```python
from build123d import *

# Parameters (mm, degrees)
SKETCH1_W            = 107
SKETCH1_H            = 36.5
BATTERY_DEPTH        = 30
CABLES_DEPTH         = 10
CABLES_DEPTH_BACK    = 5
F_1MM_EDGE_FILLETS_R = 1


with BuildPart() as part:
    # Sketch1 → Battery (new body)
    with BuildSketch(Plane(origin=(0, 0, 0), x_dir=(1, 0, 0), z_dir=(0, 1, 0))):
        Rectangle(SKETCH1_W, SKETCH1_H)
    extrude(amount=BATTERY_DEPTH)

    # Sketch2 → Cables (add, two sides: drawn at the far end of the back side and taken through both)
    with BuildSketch(Plane.ZY.offset(53.5).offset(-CABLES_DEPTH_BACK)):
        with BuildLine():
            Line((-21.25, 9.5), (-21.25, 13.5))
            ThreePointArc((-21.25, 13.5), (-19.75, 15), (-18.25, 13.5))
            Line((-18.25, 13.5), (-18.25, 9.5))
            ThreePointArc((-18.25, 9.5), (-19.75, 8), (-21.25, 9.5))
        make_face()
        with BuildLine():
            Line((17.25, 8.5), (17.25, 14.5))
            ThreePointArc((17.25, 14.5), (18.25, 15.5), (19.25, 14.5))
            Line((19.25, 14.5), (19.25, 8.5))
            ThreePointArc((19.25, 8.5), (18.25, 7.5), (17.25, 8.5))
        make_face()
    extrude(amount=CABLES_DEPTH + CABLES_DEPTH_BACK)

    # 1mm Edge Fillets
    f_1mm_edge_fillets_edges = [part.edges().sort_by_distance(p)[0] for p in [
        (0, 0, 18.25),
        (0, 0, -18.25),
        (-53.5, 0, 0),
        (0, 30, -18.25),
        (0, 30, 18.25),
        (-53.5, 30, 0),
        (53.5, 15, 18.25),
        (53.5, 30, 0),
        (53.5, 15, -18.25),
        (53.5, 0, 0),
        (-53.5, 3.75, 18.25),
        (-53.5, 22.75, 18.25),
    ]]
    fillet(f_1mm_edge_fillets_edges, radius=F_1MM_EDGE_FILLETS_R - 0.0001)  # a hair under: the kernel refuses the full size


solid = part.part
```
Geometry check sheet. Reference: the model listing, model coordinates, mm. A direction names the side the tool comes from. Coordinates: 2 decimals unless noted, no trailing zeros. Loops run counter-clockwise (first coordinate to the right, second up) from the corner with the lowest first, then second, coordinate; pieces in that order, holes last. Notation, with made-up numbers: (-28, -15.5) - (-10, -15.5) arc R24 ccw to (-10, 23.5) - close; hole circle Ø2 at (50, 70). An arc over 180 degrees is marked (long way). One line per item, written item: value. Start each with the question number.
(1) Cross-section at D-D on z = -19.75. Enter the section's corners in (x, y), plus the area to 3 significant figures.
(2) Cross-section at C-C on z = 9. Enter the section's corners in (x, y).
(3) Cross-section at B-B on y = 26.5. Enter the section's corners in (x, z).
(4) Mould release check, pull along Z, two halves, no side actions. Record for faces 5 (the flat face through (-1, 15, 18.25)), 6 (the flat face through (-58, 11, 17.25)), 7 (the flat face through (-48.5, 12, -20)): released by +Z, released by -Z, zero draft, split by the parting line, or undercut.
(5) Cross-section at A-A on x = -29.5. Enter the section's corners in (y, z).
(6) Tool access check on faces 1 (the cylindrical face through (-57.562, 7.568, 18.613)), 2 (the flat face through (-1, 30, 0)), 3 (the flat face through (-58, 12, -18.25)), 4 (the cylindrical face through (-57.562, 15.447, 18.571)). Record the directions out of +Z, -Z, +X, -X, +Y, -Y that give a thin tool (end or side, any length) a straight path to the whole face; none if there is none.
(7) Material ranges on line 1 (X direction, y = 12.5, z = 13); line 2 (Z direction, x = 20.5, y = 8), recorded low to high. Write a range as [from, to].
(8) Depth check by flat-ended pin: P1, Ø6, axis at x = -24, y = 17.5, coming from the +Z side; P2, Ø14, axis at y = 21, z = -6, coming from the -X side; P3, Ø5, axis at x = -13.5, y = 17.5, coming from the -Z side. Enter the tip coordinate at first touch or a pass-through.
Results below:
1. outline: (-63.5, 8) - (-48.5, 8) - (-48.5, 15) - (-63.5, 15) - close
1. area: 105 mm2
2. outline: (-53.5, 1) arc R1 ccw to (-52.5, 0) - (52.5, 0) arc R1 ccw to (53.5, 1) - (53.5, 29) arc R1 ccw to (52.5, 30) - (-52.5, 30) arc R1 ccw to (-53.5, 29) - close
3. outline: (-53.5, -18.25) - (52.5, -18.25) arc R1 ccw to (53.5, -17.25) - (53.5, 17.25) arc R1 ccw to (52.5, 18.25) - (-52.5, 18.25) arc R1 ccw to (-53.5, 17.25) - close
4. face 5: released by +Z
4. face 6: undercut
4. face 7: zero draft
5. outline: (0, -17.25) arc R1 ccw to (1, -18.25) - (29, -18.25) arc R1 ccw to (30, -17.25) - (30, 17.25) arc R1 ccw to (29, 18.25) - (1, 18.25) arc R1 ccw to (0, 17.25) - close
6. face 1: -X, -Y
6. face 2: +Z, -Z, +X, -X, +Y
6. face 3: -X, +Y, -Y
6. face 4: -X, +Y
7. line 1: x = [-53.5, 53.5]
7. line 2: z = [-18.25, 18.25]
8. P1: stops at z = 18.25
8. P2: stops at x = -53.5
8. P3: stops at z = -18.25
